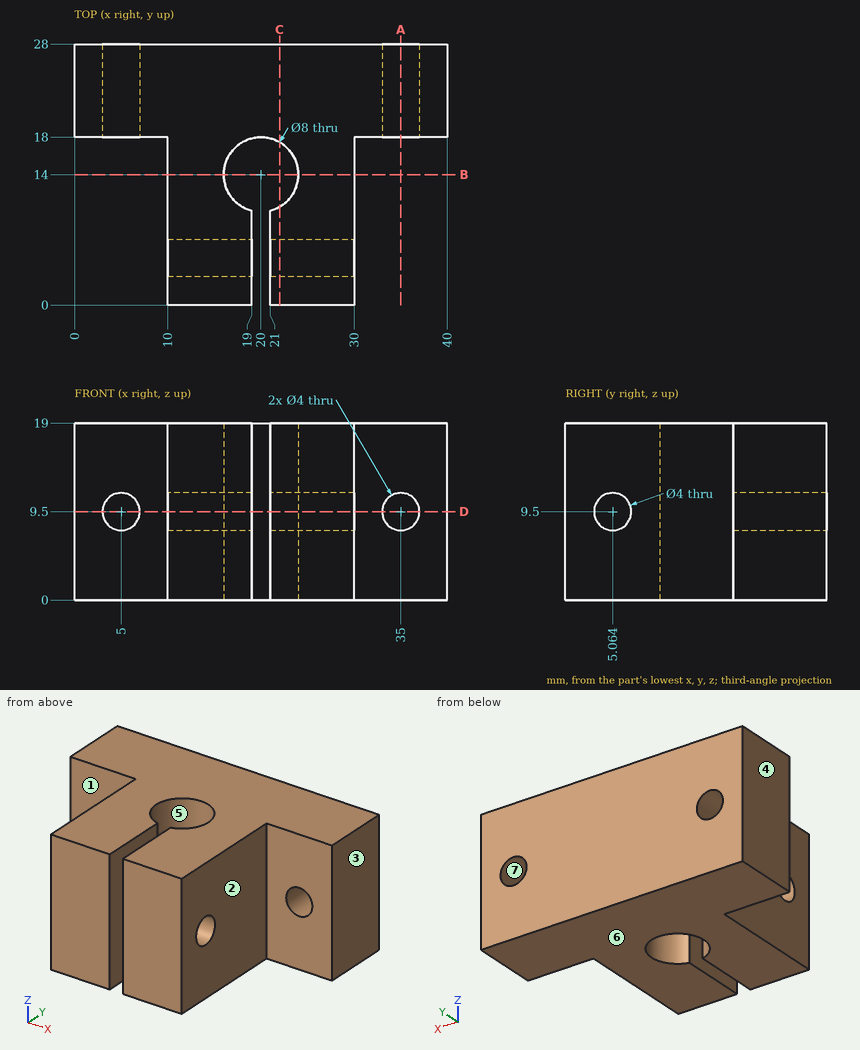
Can you work these out from the drawing? Everything is in mm from the part's minimum corner. A direction names the side the tool comes from. Round coordinates to 2 decimals unless told otherwise and drop trailing zeros. Loops run counter-clockwise (first coordinate to the right, second up) from the corner with the lowest first, then second, coordinate; pieces in that order, holes last. Notation, with made-up numbers: (26.5, 30) - (41.5, 30) arc R16 ccw to (41.5, 41) - close; hole circle Ø8 at (50.5, -16). An arc over 180 degrees is marked (long way). Answer in a Markdown table with one row per item. Add a question column.
(1) For the marked faces 1, 2 and 3, which set-ups out of +Z, -Z, +X, -X, +Y, -Y let a thin tool reach every point of the face, with its end or its side?
(2) If we mould it in two halves opening along X, with no side actions, what happens to the marked faces 4, 5, 6 and 7? For each: pulls with the +X half, pulls with the -X half, needs draft (parallel to the pull), parting line crosses it, or undercut.
(3) If we section it at B-B (y = 14): Please give me the cut outline in (x, z).
(4) If we section it at A-A (x = 35): Please give me the cut outline in (y, z).
(5) If we section it at C-C (x = 22): Please give me the cut outline in (y, z) (1 decimal), plus the area to 3 significant figures.
(6) I'm going to push flat-ended pins straight in: pin 1 (6.5 mm diameter, centred on y = 5.06, z = 9.5, fed in from +X); pin 2 (3 mm diameter, centred on x = 34.5, z = 6, fed in from -Y); pin 3 (1.5 mm diameter, centred on y = 10.5, z = 7.5, fed in from -X). Where does each tip first touch, or does it pass through?
(7) I need wall thicknesses on line 1 along X through (y, z) = (23.25, 9.5); line 2 along X through (y, z) = (7.5, 16.5); line 3 along X through (y, z) = (14, 6.5). Which ranges of each line are inside material? Lowest first, please.
(8) If we section it at D-D (z = 9.5): Please give me the cut outline in (x, y).
Model answer:
| question | item | result |
|---|---|---|
| 1 | face 1 | +Z, -Z, -X, -Y |
| 1 | face 2 | +Z, -Z, +X, -Y |
| 1 | face 3 | +Z, -Z, +X, +Y, -Y |
| 2 | face 4 | pulls with the -X half |
| 2 | face 5 | undercut |
| 2 | face 6 | needs draft |
| 2 | face 7 | undercut |
| 3 | outline | (10, 0) - (16, 0) - (16, 19) - (10, 19) - close; (24, 0) - (30, 0) - (30, 19) - (24, 19) - close |
| 4 | outline | (18, 0) - (28, 0) - (28, 7.5) - (18, 7.5) - close; (18, 11.5) - (28, 11.5) - (28, 19) - (18, 19) - close |
| 5 | outline | (0, 0) - (10.5, 0) - (10.5, 19) - (0, 19) - close; (17.5, 0) - (28, 0) - (28, 19) - (17.5, 19) - close; hole circle Ø4 at (5.1, 9.5) |
| 5 | area | 388 mm² |
| 6 | pin 1 | stops at x = 30 |
| 6 | pin 2 | stops at y = 18 |
| 6 | pin 3 | stops at x = 10 |
| 7 | line 1 | x = 0 to 3, 7 to 33, 37 to 40 |
| 7 | line 2 | x = 10 to 19, 21 to 30 |
| 7 | line 3 | x = 10 to 16, 24 to 30 |
| 8 | outline | (0, 18) - (3, 18) - (3, 28) - (0, 28) - close; (7, 18) - (10, 18) - (10, 7.06) - (19, 7.06) - (19, 10.13) arc R4 cw (long way) to (21, 10.13) - (21, 7.06) - (30, 7.06) - (30, 18) - (33, 18) - (33, 28) - (7, 28) - close; (10, 0) - (19, 0) - (19, 3.06) - (10, 3.06) - close; (21, 0) - (30, 0) - (30, 3.06) - (21, 3.06) - close; (37, 18) - (40, 18) - (40, 28) - (37, 28) - close |
